Work out the finished part from the listing and answer in its coordinate system (mm). A direction names the side the tool comes from. Round coordinates to 2 decimals unless told otherwise and drop trailing zeros. Order: outer loops, then holes, each group sorted by start corner. A loop starts at its lowest first (then second) coordinate and runs counter-clockwise, first axis right, second up. Notation, with made-up numbers: (-20, 85) - (11, 85) arc R20 ccw to (11, 89) - close; hole circle Ø2 at (40, 10.5). An arc over 180 degrees is marked (long way). Put each result on its own line as item: value.
```python
from build123d import *

# Parameters (mm, degrees)
CBORE_FOR_M2_5_SHCS1_AT_2_COUNT = 2
CBORE_FOR_M2_5_SHCS1_AT_2_PITCH = 8.419035512
CBORE_FOR_M2_5_SHCS1_AT_3_COUNT = 2
CBORE_FOR_M2_5_SHCS1_AT_3_PITCH = 20.325349715
CBORE_FOR_M2_5_SHCS1_AT_4_COUNT = 2
CBORE_FOR_M2_5_SHCS1_AT_4_PITCH = 22
CBORE_FOR_M2_5_SHCS1_AT_5_COUNT = 2
CBORE_FOR_M2_5_SHCS1_AT_5_PITCH = 20.325349715
CBORE_FOR_M2_5_SHCS1_AT_6_COUNT = 2
CBORE_FOR_M2_5_SHCS1_AT_6_PITCH = 8.419035512
SKETCH6_W                       = 0.75
SKETCH6_H                       = 1.5
SKETCH8_W                       = 4
SKETCH8_H                       = 4
BOSS_EXTRUDE1_DEPTH             = 12


with BuildPart() as part:
    # Sketch1 → Revolve1 (revolve)
    with BuildSketch(Plane(origin=(0, 0, 0), x_dir=(1, 0, 0), z_dir=(0, 1, 0))):
        Polygon((0, 24), (0, 3), (6, 3), (6, 0), (14, 0), (14, 8), (8.5, 8), (8.5, 24), align=None)
    revolve(axis=Axis((0, 0, 25.877450995), (0, 0, -1)))

    # Sketch4 → CBORE for M2.5 SHCS1 (revolve, cut)
    with BuildSketch(Plane(origin=(-11, 0, -8), x_dir=(0, 1, 0), z_dir=(1, 0, 0))):
        Polygon((0, 0), (0, 8), (1.45, 8), (1.45, 2.5), (2.75, 2.5), (2.75, 0.025), (2.775, 0), align=None)
    cbore_for_m2_5_shcs1 = revolve(axis=Axis((-11, 0, -14.35), (0, 0, 1)), mode=Mode.SUBTRACT)

    # CBORE for M2.5 SHCS1 at 2: CBORE for M2.5 SHCS1 ×2
    with Locations(*[Vector(0.38268343236508967, 0.9238795325112867, 0) * (i * CBORE_FOR_M2_5_SHCS1_AT_2_PITCH) for i in range(1, CBORE_FOR_M2_5_SHCS1_AT_2_COUNT)]):
        add(cbore_for_m2_5_shcs1, mode=Mode.SUBTRACT)

    # CBORE for M2.5 SHCS1 at 3: CBORE for M2.5 SHCS1 ×2
    with Locations(*[Vector(0.9238795325112867, 0.3826834323650897, 0) * (i * CBORE_FOR_M2_5_SHCS1_AT_3_PITCH) for i in range(1, CBORE_FOR_M2_5_SHCS1_AT_3_COUNT)]):
        add(cbore_for_m2_5_shcs1, mode=Mode.SUBTRACT)

    # CBORE for M2.5 SHCS1 at 4: CBORE for M2.5 SHCS1 ×2
    with Locations(*[(i * CBORE_FOR_M2_5_SHCS1_AT_4_PITCH, 0, 0) for i in range(1, CBORE_FOR_M2_5_SHCS1_AT_4_COUNT)]):
        add(cbore_for_m2_5_shcs1, mode=Mode.SUBTRACT)

    # CBORE for M2.5 SHCS1 at 5: CBORE for M2.5 SHCS1 ×2
    with Locations(*[Vector(0.9238795325112867, -0.38268343236508984, 0) * (i * CBORE_FOR_M2_5_SHCS1_AT_5_PITCH) for i in range(1, CBORE_FOR_M2_5_SHCS1_AT_5_COUNT)]):
        add(cbore_for_m2_5_shcs1, mode=Mode.SUBTRACT)

    # CBORE for M2.5 SHCS1 at 6: CBORE for M2.5 SHCS1 ×2
    with Locations(*[Vector(0.38268343236508967, -0.9238795325112868, 0) * (i * CBORE_FOR_M2_5_SHCS1_AT_6_PITCH) for i in range(1, CBORE_FOR_M2_5_SHCS1_AT_6_COUNT)]):
        add(cbore_for_m2_5_shcs1, mode=Mode.SUBTRACT)

    # Sketch6 → Cut-Revolve1 (revolve, cut)
    with BuildSketch(Plane(origin=(0, 0, 0), x_dir=(1, 0, 0), z_dir=(0, 1, 0))):
        with Locations((8.125, 20.75)):
            Rectangle(SKETCH6_W, SKETCH6_H)
    revolve(axis=Axis((0, 0, 6.058618002), (0, 0, -1)), mode=Mode.SUBTRACT)

    # Sketch8 → Boss-Extrude1 (add)
    with BuildSketch(Plane.XY.offset(-20)):
        with Locations((0, 8)):
            Rectangle(SKETCH8_W, SKETCH8_H)
    extrude(amount=BOSS_EXTRUDE1_DEPTH)


solid = part.part
```
1) For a pull along X with two mould halves and no side action, classify faces 4 (the flat face through (-3, 6, 0)), 5 (the cylindrical face through (4.57, -7.167, -22.768)), 6 (the flat face through (12.2, -1.2, -5.5)) as pulls with the +X half, pulls with the -X half, needs draft (parallel to the pull), parting line crosses it, or undercut.
Findings below:
face 4: needs draft
face 5: parting line crosses it
face 6: undercut
2) Given pin 1 Ø2 at (x, z) = (6.5, -5.5) entering from -Y; pin 2 Ø4.5 at (x, y) = (7.78, 7.78) entering from -Z; pin 3 Ø8 at (y, z) = (5, -18) entering from +X, each flat-ended and moving along its own axis, determine where each tip first touches the part or whether it passes through.
Findings below:
pin 1: stops at y = -12.87
pin 2: stops at z = -5.5
pin 3: stops at x = 8.44
3) A cutting plane is placed at A-A on x = -11. Write down the section's boundary in (y, z) (3 decimals), then the cut area to 3 significant figures.
Findings below:
outline: (-8.66, -8) - (-2.775, -8) - (-2.75, -7.975) - (-2.75, -5.5) - (-1.45, -5.5) - (-1.45, 0) - (-8.66, 0) - close; (1.45, -5.5) - (2.75, -5.5) - (2.75, -7.975) - (2.775, -8) - (8.66, -8) - (8.66, 0) - (1.45, 0) - close
area: 109 mm2
4) Straight lines are drawn through the part: L1, parallel to Z at x = 1, y = -7.75; L2, parallel to Z at x = -11, y = -5.5; L3, parallel to X at y = 2, z = -6.5. For each, find the intervals that lie inside material, in ascending order. Write a range as from..to.
Findings below:
L1: z = -24..-21.5, -20..0
L2: z = -8..0
L3: x = -13.86..-12.89, -9.11..9.11, 12.89..13.86
5) A cutting plane is placed at C-C on y = 0. Give the number of separate pieces and of enclosed holes in the cut face, then the cut area to 3 significant figures.
Findings below:
separate pieces: 3
enclosed holes: 0
area: 398 mm2
6) A cutting plane is placed at B-B on z = -5. Write down the section's boundary in (x, y).
Findings below:
outline: circle Ø28 at (0, 0); hole circle Ø2.9 at (-11, 0); hole circle Ø2.9 at (-7.78, -7.78); hole circle Ø2.9 at (-7.78, 7.78); hole circle Ø2.9 at (7.78, -7.78); hole circle Ø2.9 at (7.78, 7.78); hole circle Ø2.9 at (11, 0)
7) For faces 1 (the flat face through (-8, -2, -21.5)), 2 (the cylindrical face through (6.34, -7.97, -2.79)), 3 (the flat face through (0, 0, -3)), determine the directions among +Z, -Z, +X, -X, +Y, -Y from which every point of the face is accessible in a straight line to the end or side of a thin tool.
Findings below:
face 1: none
face 2: +Z, -Z
face 3: +Z
8) A cutting plane is placed at D-D on x = 0. Write down the section's boundary in (y, z), then the cut area to 3 significant figures.
Findings below:
outline: (-14, -8) - (-8.5, -8) - (-8.5, -20) - (-7.75, -20) - (-7.75, -21.5) - (-8.5, -21.5) - (-8.5, -24) - (8.5, -24) - (8.5, -21.5) - (7.75, -21.5) - (7.75, -20) - (10, -20) - (10, -8) - (14, -8) - (14, 0) - (6, 0) - (6, -3) - (-6, -3) - (-6, 0) - (-14, 0) - close
area: 476 mm2
